Part model, mm, in its own coordinate system. Face numbers are marked on the shaded views. A direction names the side the tool comes from. Coordinates: 2 decimals unless noted, no trailing zeros. Order: outer loops, then holes, each group sorted by start corner. A loop starts at its lowest first (then second) coordinate and runs counter-clockwise, first axis right, second up.
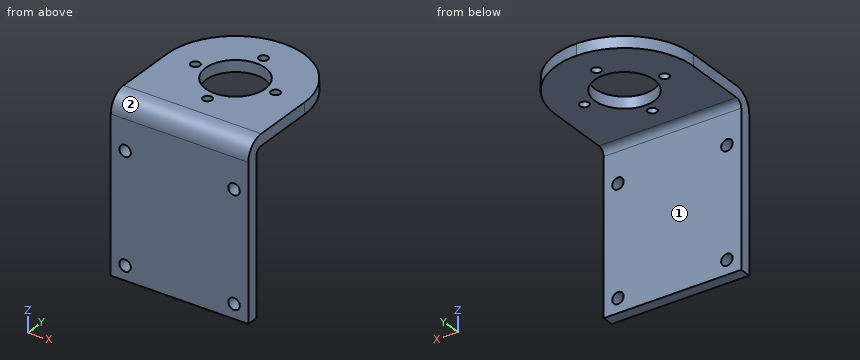
from build123d import *

# Parameters (mm, degrees)
SKETCH_10_W                      = 60
SKETCH_10_H                      = 60
SM_BASE_FLANGE_2_DEPTH           = 5
SM_EDGE_FLANGE_2_STRIP_W         = 26
SM_EDGE_FLANGE_2_STRIP_H         = 5
SM_EDGE_FLANGE_2_STRIP_CUT_DEPTH = 60
SM_EDGE_FLANGE_2_DEPTH           = 60
SKETCH_19_R                      = 2
SKETCH_19_R_2                    = 13
CUT_EXTRUDE_2_DEPTH              = 5
CUT_EXTRUDE_START                = -30
SKETCH_28_R                      = 2.5
CUT_EXTRUDE_4_DEPTH              = 5
CUT_EXTRUDE_5_DEPTH              = 5


# Sheet-metal steps are written as plain solids
with BuildPart() as part:
    # 草图10 → 基体-法兰2 (new body)
    with BuildSketch(Plane.XY):
        Rectangle(SKETCH_10_W, SKETCH_10_H)
    extrude(amount=-SM_BASE_FLANGE_2_DEPTH)

    # 边线-法兰2 strip (across the edge) → 边线-法兰2 strip cut (cut)
    with BuildSketch(Plane(origin=(30, -30, -5), x_dir=(0, 1, 0), z_dir=(-1, 0, 0))):
        with Locations((-10, -2.5)):
            Rectangle(SM_EDGE_FLANGE_2_STRIP_W, SM_EDGE_FLANGE_2_STRIP_H)
    extrude(amount=SM_EDGE_FLANGE_2_STRIP_CUT_DEPTH, mode=Mode.SUBTRACT)

    # 边线-法兰2 section (across the edge) → 边线-法兰2 (add)
    with BuildSketch(Plane(origin=(30, -30, -5), x_dir=(0, 1, 0), z_dir=(-1, 0, 0))):
        with BuildLine():
            Line((-5, 3), (-5, 70))
            Line((-5, 70), (0, 70))
            Line((0, 70), (0, 3))
            ThreePointArc((0, 3), (0.878679656, 0.878679656), (3, 0))
            Line((3, 0), (3, -5))
            ThreePointArc((3, -5), (-2.656854249, -2.656854249), (-5, 3))
        make_face()
    extrude(amount=SM_EDGE_FLANGE_2_DEPTH)

    # 草图19 → 切除-拉伸2 (cut)
    with BuildSketch(Plane.XY):
        with Locations(Location((-17.5, 0, 0), (0, 0, 180))):
            Circle(SKETCH_19_R)
        with Locations(Location((17.5, 0, 0), (0, 0, 180))):
            Circle(SKETCH_19_R)
        with Locations(Location((0, 17.5, 0), (0, 0, 180))):
            Circle(SKETCH_19_R)
        with Locations(Location((0, -17.5, 0), (0, 0, 180))):
            Circle(SKETCH_19_R)
        with Locations(Location((0, 0, 0), (0, 0, 180))):
            Circle(SKETCH_19_R_2)
    extrude(amount=-CUT_EXTRUDE_2_DEPTH, mode=Mode.SUBTRACT)

    # 草图28 → 切除-拉伸4 (cut)
    with BuildSketch(Plane(origin=(0, 0, 0), x_dir=(1, 0, 0), z_dir=(0, 1, 0)).offset(CUT_EXTRUDE_START)):
        with Locations(Location((-23.75, 21.25, 0), (0, 0, 90))):
            Circle(SKETCH_28_R)
        with Locations(Location((-23.75, 68.75, 0), (0, 0, 90))):
            Circle(SKETCH_28_R)
        with Locations(Location((23.75, 68.75, 0), (0, 0, 90))):
            Circle(SKETCH_28_R)
        with Locations(Location((23.75, 21.25, 0), (0, 0, 90))):
            Circle(SKETCH_28_R)
    extrude(amount=-CUT_EXTRUDE_4_DEPTH, mode=Mode.SUBTRACT)

    # 草图29 → 切除-拉伸5 (cut)
    with BuildSketch(Plane.XY):
        with BuildLine():
            ThreePointArc((-30, 0), (-21.213203436, 21.213203436), (0, 30))
            Line((0, 30), (-30, 30))
            Line((-30, 30), (-30, 0))
        make_face()
        with BuildLine():
            Line((30, 30), (0, 30))
            ThreePointArc((0, 30), (21.213203436, 21.213203436), (30, 0))
            Line((30, 0), (30, 30))
        make_face()
    extrude(amount=-CUT_EXTRUDE_5_DEPTH, mode=Mode.SUBTRACT)


solid = part.part
Q1. Which spindle directions (+Z, -Z, +X, -X, +Y, -Y) get a long thin tool onto all of the face, cutting with end or side? Do the marked faces 1 and 2. Say none if no direction does.
Results list:
face 1: -Z, +X, -X, +Y
face 2: +Z, +X, -X, -Y
Q2. Cut at D-D on y = 4.5. Write the cut outline in (x, z), and give its area (3 significant figures).
Results list:
outline: (-29.66, -5) - (-12.2, -5) - (-12.2, 0) - (-29.66, 0) - close; (12.2, -5) - (29.66, -5) - (29.66, 0) - (12.2, 0) - close
area: 175 mm2
Q3. Cut at B-B on x = 22.5. Write the cut outline in (y, z), and give its area (3 significant figures).
Results list:
outline: (-35, -75) - (-30, -75) - (-30, -70.92) - (-35, -70.92) - close; (-35, -66.58) - (-30, -66.58) - (-30, -23.42) - (-35, -23.42) - close; (-35, -19.08) - (-30, -19.08) - (-30, -8) arc R3 cw to (-27, -5) - (19.84, -5) - (19.84, 0) - (-27, 0) arc R8 ccw to (-35, -8) - close
area: 569 mm2
Q4. Cut at C-C on x = -17.5. Write the cut outline in (y, z), and give its area (3 significant figures).
Results list:
outline: (-35, -75) - (-30, -75) - (-30, -8) arc R3 cw to (-27, -5) - (-2, -5) - (-2, 0) - (-27, 0) arc R8 ccw to (-35, -8) - close; (2, -5) - (24.37, -5) - (24.37, 0) - (2, 0) - close
area: 615 mm2
Q5. Wall check: line 1 along X through (y, z) = (-31.5, -21.25); line 2 along Z through (x, y) = (23.75, -32.3); line 3 along Y through (x, z) = (0, -3.85). Give the ranges that are in metal, low to high.
Results list:
line 1: x = -30 to -26.25, -21.25 to 21.25, 26.25 to 30
line 2: z = -75 to -71.25, -66.25 to -23.75, -18.75 to -2.01
line 3: y = -33.84 to -19.5, -15.5 to -13, 13 to 15.5, 19.5 to 30
Q6. Cut at A-A on y = -17.5. Write the cut outline in (x, z).
Results list:
outline: (-30, -5) - (-2, -5) - (-2, 0) - (-30, 0) - close; (2, -5) - (30, -5) - (30, 0) - (2, 0) - close
Q7. Pin check, flat tips, straight feed: pin 1 Ø5 at (y, z) = (-24, -8.5) entering from -X; pin 2 Ø6.5 at (x, y) = (17.5, 0) entering from -Z; pin 3 Ø3 at (x, z) = (-23, -62.5) entering from +Y; pin 4 Ø1 at (x, y) = (18, -20) entering from +Z. Stop position of each tip, or through.
Results list:
pin 1: passes through
pin 2: stops at z = -5
pin 3: stops at y = -30
pin 4: stops at z = 0
